```python
from build123d import *

# Parameters (mm, degrees)
SKETCH1_R           = 23
SKETCH1_R_2         = 10
BOSS_EXTRUDE1_DEPTH = 4
SKETCH2_R           = 20
SKETCH2_R_2         = 10
SKETCH2_R_3         = 2
BOSS_EXTRUDE2_DEPTH = 30


with BuildPart() as part:
    # Sketch1 → Boss-Extrude1 (new body)
    with BuildSketch(Plane.XY):
        Circle(SKETCH1_R)
        Circle(SKETCH1_R_2, mode=Mode.SUBTRACT)
    extrude(amount=BOSS_EXTRUDE1_DEPTH)

    # Sketch2 → Boss-Extrude2 (add)
    with BuildSketch(Plane.XY.offset(4)):
        Circle(SKETCH2_R)
        Circle(SKETCH2_R_2, mode=Mode.SUBTRACT)
        with Locations((0, 15)):
            Circle(SKETCH2_R_3, mode=Mode.SUBTRACT)
        with Locations((15, 0)):
            Circle(SKETCH2_R_3, mode=Mode.SUBTRACT)
        with Locations((0, -15)):
            Circle(SKETCH2_R_3, mode=Mode.SUBTRACT)
        with Locations((-15, 0)):
            Circle(SKETCH2_R_3, mode=Mode.SUBTRACT)
    extrude(amount=BOSS_EXTRUDE2_DEPTH)


solid = part.part
```
Part model, mm, in its own coordinate system. A direction names the side the tool comes from. Round coordinates to 2 decimals unless told otherwise and drop trailing zeros. Order: outer loops, then holes, each group sorted by start corner. A loop starts at its lowest first (then second) coordinate and runs counter-clockwise, first axis right, second up. Notation, with made-up numbers: M 78,50 L 85,50 A13 ccw 85,56 Z; hole C -5.75,62 d8. An arc over 180 degrees is marked long. Answer in a Markdown table with one row per item. Add a question column.
Q1. Mould opens along X. For faces 1 (the face through (-7, 19, 4)), 2 (the face through (13.4, -1.2, 18.8)), 3 (the face through (-4.336, -19.524, 18.79)) say: +X half, -X half, draft (parallel to the pull), parting line (faces both ways), or undercut.
Q2. Cut at B-B on z = 17. Give the cut face in (x, y), and give its area (3 significant figures).
Q3. Pin check, flat tips, straight feed: pin 1 (3.5 mm diameter, centred on x = 0, y = -15, fed in from +Z); pin 2 (8 mm diameter, centred on x = -14.5, z = 20, fed in from -Y); pin 3 (8 mm diameter, centred on y = -6.5, z = 11, fed in from -X); pin 4 (12 mm diameter, centred on x = 0, y = 0, fed in from +Z). Stop position of each tip, or through.
Q4. 3-axis set-ups, long thin cutter, end or side, ignore diameter. For faces 4 (the face through (-16.6, -1.2, 18.8)), 5 (the face through (10, -5, 0)): which of +Z, -Z, +X, -X, +Y, -Y reach the whole face in a straight line?
Q5. Wall check: L1, parallel to Y at x = 0, z = 15; L2, parallel to Z at x = 6, y = 20.5; L3, parallel to X at y = 5.5, z = 23. Give the ranges that are in metal, low to high. Write a range as from..to.
Q6. Cut at A-A on y = 0. Give the cut face in (x, z), and give its area (3 significant figures).
Q7. Cut at D-D on y = 15. Give the cut face in (x, z).
Established:
| question | item | result |
|---|---|---|
| 1 | face 1 | draft |
| 1 | face 2 | undercut |
| 1 | face 3 | parting line |
| 2 | outline | C 0,0 d40; hole C -15,0 d4; hole C 0,0 d20; hole C 0,-15 d4; hole C 0,15 d4; hole C 15,0 d4 |
| 2 | area | 892 mm2 |
| 3 | pin 1 | stops at z = 4 |
| 3 | pin 2 | stops at y = -17.02 |
| 3 | pin 3 | stops at x = -19.84 |
| 3 | pin 4 | passes through |
| 4 | face 4 | +Z |
| 4 | face 5 | -Z, +X, -X, +Y, -Y |
| 5 | L1 | y = -20..-17, -13..-10, 10..13, 17..20 |
| 5 | L2 | z = 0..4 |
| 5 | L3 | x = -19.23..-8.35, 8.35..19.23 |
| 6 | outline | M -23,0 L -10,0 L -10,34 L -13,34 L -13,4 L -17,4 L -17,34 L -20,34 L -20,4 L -23,4 Z; M 10,0 L 23,0 L 23,4 L 20,4 L 20,34 L 17,34 L 17,4 L 13,4 L 13,34 L 10,34 Z |
| 6 | area | 464 mm2 |
| 7 | outline | M -17.44,0 L 17.44,0 L 17.44,4 L 13.23,4 L 13.23,34 L 2,34 L 2,4 L -2,4 L -2,34 L -13.23,34 L -13.23,4 L -17.44,4 Z |
